```python
from build123d import *

# Parameters (mm, degrees)
SKETCH1_R           = 1.75
BOSS_EXTRUDE1_DEPTH = 2.5


with BuildPart() as part:
    # Sketch1 → Boss-Extrude1 (new body)
    with BuildSketch(Plane.XY):
        with BuildLine():
            Line((0, -17.5), (0, 17.5))
            Line((0, 17.5), (5, 17.5))
            Line((5, 17.5), (5, 9.554775034))
            ThreePointArc((5, 9.554775034), (5.732233047, 7.787008081), (7.5, 7.054775034))
            Line((7.5, 7.054775034), (17.5, 7.054775034))
            ThreePointArc((17.5, 7.054775034), (19.267766953, 7.787008081), (20, 9.554775034))
            Line((20, 9.554775034), (20, 17.5))
            Line((20, 17.5), (25, 17.5))
            Line((25, 17.5), (25, 9.554775034))
            ThreePointArc((25, 9.554775034), (25.732233047, 7.787008081), (27.5, 7.054775034))
            Line((27.5, 7.054775034), (33.501638743, 7.054775034))
            ThreePointArc((33.501638743, 7.054775034), (34.562298915, 6.615435205), (35.001638743, 5.554775034))
            Line((35.001638743, 5.554775034), (35.001638743, 4.554775034))
            ThreePointArc((35.001638743, 4.554775034), (35.440978571, 3.494114862), (36.501638743, 3.054775034))
            Line((36.501638743, 3.054775034), (47, 3.054775034))
            ThreePointArc((47, 3.054775034), (49.121320344, 2.176095377), (50, 0.054775034))
            Line((50, 0.054775034), (50, -0.054775034))
            ThreePointArc((50, -0.054775034), (49.121320344, -2.176095377), (47, -3.054775034))
            Line((47, -3.054775034), (36.501638743, -3.054775034))
            ThreePointArc((36.501638743, -3.054775034), (35.440978571, -3.494114862), (35.001638743, -4.554775034))
            Line((35.001638743, -4.554775034), (35.001638743, -5.554775034))
            ThreePointArc((35.001638743, -5.554775034), (34.562298915, -6.615435205), (33.501638743, -7.054775034))
            Line((33.501638743, -7.054775034), (27.5, -7.054775034))
            ThreePointArc((27.5, -7.054775034), (25.732233047, -7.787008081), (25, -9.554775034))
            Line((25, -9.554775034), (25, -17.5))
            Line((25, -17.5), (20, -17.5))
            Line((20, -17.5), (20, -9.554775034))
            ThreePointArc((20, -9.554775034), (19.267766953, -7.787008081), (17.5, -7.054775034))
            Line((17.5, -7.054775034), (7.5, -7.054775034))
            ThreePointArc((7.5, -7.054775034), (5.732233047, -7.787008081), (5, -9.554775034))
            Line((5, -9.554775034), (5, -17.5))
            Line((5, -17.5), (0, -17.5))
        make_face()
        with Locations((43.591641256, 0)):
            Circle(SKETCH1_R, mode=Mode.SUBTRACT)
        with BuildLine():
            Line((7.5, 1), (17.5, 1))
            ThreePointArc((17.5, 1), (18.5, 0), (17.5, -1))
            Line((17.5, -1), (7.5, -1))
            ThreePointArc((7.5, -1), (6.5, 0), (7.5, 1))
        make_face(mode=Mode.SUBTRACT)
        with BuildLine():
            Line((21.935113123, 1.8014467), (38.399570766, 1.8014467))
            ThreePointArc((38.399570766, 1.8014467), (40.201017466, 0), (38.399570766, -1.8014467))
            Line((38.399570766, -1.8014467), (21.935113123, -1.8014467))
            ThreePointArc((21.935113123, -1.8014467), (20.133666423, 0), (21.935113123, 1.8014467))
        make_face(mode=Mode.SUBTRACT)
    extrude(amount=BOSS_EXTRUDE1_DEPTH)


solid = part.part
```
Work out the finished part from the listing and answer in its coordinate system (mm). A direction names the side the tool comes from. Coordinates: 2 decimals unless noted, no trailing zeros. Write each loop counter-clockwise with the first axis right and the second up, starting at its lowest first coordinate (ties: lowest second). Pieces come first, ordered by that corner, then holes. Notation, with made-up numbers: (46.25, 27.25) - (89.25, 27.25) arc R27 ccw to (89.25, 63.25) - close; hole circle Ø7 at (-34.5, -38.75). An arc over 180 degrees is marked (long way). Answer as a JSON object with one key per item and string values.
Q1. For a pull along X with two mould halves and no side action, classify faces 1 (the flat face through (20, 13, 1)), 2 (the cylindrical face through (34.574, -6.604, 1.232)), 3 (the cylindrical face through (5.75, -7.77, 1.23)), 4 (the flat face through (42, -3.055, 1)) as pulls with the +X half, pulls with the -X half, needs draft (parallel to the pull), parting line crosses it, or undercut.
Results list:
{"face 1": "undercut", "face 2": "pulls with the +X half", "face 3": "undercut", "face 4": "needs draft"}
Q2. Given pin 1 Ø0.8 at (x, z) = (13.5, 1) entering from -Y; pin 2 Ø0.8 at (x, z) = (29.5, 1.5) entering from +Y; pin 3 Ø0.8 at (y, z) = (5, 1.5) entering from +X; pin 4 Ø3 at (x, y) = (43.59, 0) entering from -Z, each flat-ended and moving along its own axis, determine where each tip first touches the part or whether it passes through.
Results list:
{"pin 1": "stops at y = -7.05", "pin 2": "stops at y = 7.05", "pin 3": "stops at x = 35", "pin 4": "passes through"}
Q3. Which of the six approach directions +Z, -Z, +X, -X, +Y, -Y give full straight-line access (tool end or side, diameter ignored) to faces 5 (the cylindrical face through (19.29, -7.81, 1.23)), 6 (the flat face through (5, 14, 1)), 7 (the flat face through (31, -7.055, 1)), 8 (the flat face through (35.002, 5, 1)), 9 (the cylindrical face through (18.5, 0, 1.2))?
Results list:
{"face 5": "+Z, -Z, -Y", "face 6": "+Z, -Z, +Y", "face 7": "+Z, -Z, +X, -Y", "face 8": "+Z, -Z, +X, +Y", "face 9": "+Z, -Z"}
Q4. Find section C-C (z = 1.6). State how many separate pieces and enclosed holes the cut face has, plus the area to 3 significant figures.
Results list:
{"separate pieces": "1", "enclosed holes": "3", "area": "696 mm^2"}
Q5. Find section A-A (x = 17). Write down the section's boundary in (y, z).
Results list:
{"outline": "(-7.05, 0) - (-1, 0) - (-1, 2.5) - (-7.05, 2.5) - close; (1, 0) - (7.05, 0) - (7.05, 2.5) - (1, 2.5) - close"}
Q6. Consider L1, parallel to Y at x = 37, z = 1.9; L2, parallel to X at y = 14.5, z = 0.1; L3, parallel to Y at x = 29, z = 2.05. Determine where each line is inside the solid, lowest interval first. Write a range as from..to.
Results list:
{"L1": "y = -3.05..-1.8, 1.8..3.05", "L2": "x = 0..5, 20..25", "L3": "y = -7.05..-1.8, 1.8..7.05"}
Q7. Find section B-B (y = 14.5). Write down the section's boundary in (x, z).
Results list:
{"outline": "(0, 0) - (5, 0) - (5, 2.5) - (0, 2.5) - close; (20, 0) - (25, 0) - (25, 2.5) - (20, 2.5) - close"}
